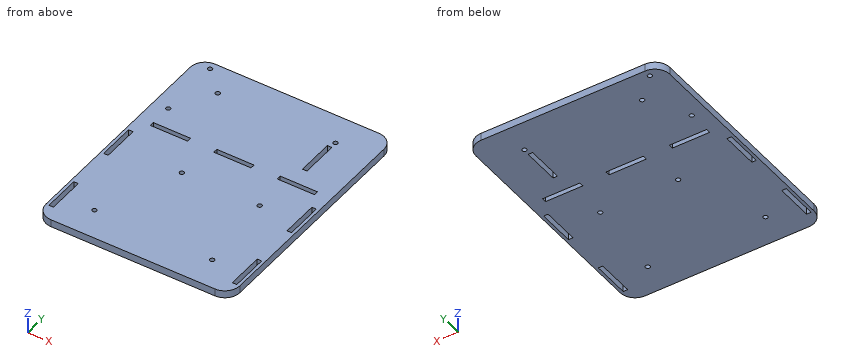
from build123d import *

# Parameters (mm, degrees)
RESSALTO_EXTRUS_O1_DEPTH = 5
ESBO_O2_R                = 1.5
CORTE_EXTRUS_O1_DEPTH    = 5
ESBO_O3_R                = 1.5
CORTE_EXTRUS_O2_DEPTH    = 6
ESBO_O6_W                = 3
ESBO_O6_H                = 25
ESBO_O6_W_2              = 25
ESBO_O6_H_2              = 3
CORTE_EXTRUS_O4_DEPTH    = 6
ESBO_O8_R                = 1.5
CORTE_EXTRUS_O6_DEPTH    = 10
ESBO_O9_W                = 3
ESBO_O9_H                = 25
CORTE_EXTRUS_O7_DEPTH    = 10


with BuildPart() as part:
    # Esboço1 → Ressalto-extrusão1 (new body)
    with BuildSketch(Plane.XY):
        with BuildLine():
            Line((-49.217119449, -36.393854661), (60.782880551, -36.393854661))
            ThreePointArc((60.782880551, -36.393854661), (67.853948363, -33.464922473), (70.782880551, -26.393854661))
            Line((70.782880551, -26.393854661), (70.782880551, 118.606145339))
            ThreePointArc((70.782880551, 118.606145339), (67.853948363, 125.67721315), (60.782880551, 128.606145339))
            Line((60.782880551, 128.606145339), (-49.217119449, 128.606145339))
            ThreePointArc((-49.217119449, 128.606145339), (-56.288187261, 125.67721315), (-59.217119449, 118.606145339))
            Line((-59.217119449, 118.606145339), (-59.217119449, -26.393854661))
            ThreePointArc((-59.217119449, -26.393854661), (-56.288187261, -33.464922473), (-49.217119449, -36.393854661))
        make_face()
    extrude(amount=RESSALTO_EXTRUS_O1_DEPTH)

    # Esboço2 → Corte-extrusão1 (cut)
    with BuildSketch(Plane(origin=(0, 0, 0), x_dir=(-1, 0, 0), z_dir=(0, 0, -1))):
        with Locations((33.717119449, -15.893854661)):
            Circle(ESBO_O2_R)
        with Locations((33.717119449, 108.106145339)):
            Circle(ESBO_O2_R)
        with Locations((-45.282880551, -15.893854661)):
            Circle(ESBO_O2_R)
        with Locations((-45.282880551, 108.106145339)):
            Circle(ESBO_O2_R)
    extrude(amount=-CORTE_EXTRUS_O1_DEPTH, mode=Mode.SUBTRACT)

    # Esboço3 → Corte-extrusão2 (cut, through all)
    with BuildSketch(Plane(origin=(0, 0, 0), x_dir=(-1, 0, 0), z_dir=(0, 0, -1))):
        with Locations((49.217119449, 123.606145339)):
            Circle(ESBO_O3_R)
        with Locations((49.217119449, 81.556145339)):
            Circle(ESBO_O3_R)
    extrude(amount=-CORTE_EXTRUS_O2_DEPTH, mode=Mode.SUBTRACT)

    # Esboço6 → Corte-extrusão4 (cut, through all)
    with BuildSketch(Plane(origin=(0, 0, 0), x_dir=(-1, 0, 0), z_dir=(0, 0, -1))):
        with Locations((-67.282880551, -13.893854661)):
            Rectangle(ESBO_O6_W, ESBO_O6_H)
        with Locations((-67.282880551, 41.106145339)):
            Rectangle(ESBO_O6_W, ESBO_O6_H)
        with Locations((-48.282880551, 65.106145339)):
            Rectangle(ESBO_O6_W_2, ESBO_O6_H_2)
        with Locations((36.717119449, 65.106145339)):
            Rectangle(ESBO_O6_W_2, ESBO_O6_H_2)
        with Locations((55.717119449, 41.106145339)):
            Rectangle(ESBO_O6_W, ESBO_O6_H)
        with Locations((55.717119449, -13.893854661)):
            Rectangle(ESBO_O6_W, ESBO_O6_H)
        with Locations((-5.782880551, 65.106145339)):
            Rectangle(ESBO_O6_W_2, ESBO_O6_H_2)
    extrude(amount=-CORTE_EXTRUS_O4_DEPTH, mode=Mode.SUBTRACT)

    # Esboço8 → Corte-extrusão6 (cut)
    with BuildSketch(Plane.XY.offset(5)):
        with Locations((-11.447119449, 38.606145339)):
            Circle(ESBO_O8_R)
        with Locations((40.782880551, 38.606145339)):
            Circle(ESBO_O8_R)
    extrude(amount=-CORTE_EXTRUS_O6_DEPTH, mode=Mode.SUBTRACT)

    # Esboço9 → Corte-extrusão7 (cut)
    with BuildSketch(Plane(origin=(0, 0, 0), x_dir=(-1, 0, 0), z_dir=(0, 0, -1))):
        with Locations((-44.282880551, 91.106145339)):
            Rectangle(ESBO_O9_W, ESBO_O9_H)
    extrude(amount=-CORTE_EXTRUS_O7_DEPTH, mode=Mode.SUBTRACT)


solid = part.part
Work out the finished part from the listing and answer in its coordinate system (mm). Round coordinates to 2 decimals unless told otherwise and drop trailing zeros. Write each loop counter-clockwise with the first axis right and the second up, starting at its lowest first coordinate (ties: lowest second). Pieces come first, ordered by that corner, then holes.
1) A cutting plane is placed at B-B (x = 0). Give the vertices of the cut face in (y, z), plus the area to 3 significant figures.
2) A cutting plane is placed at C-C (z = 2.85). Give the number of separate pieces and of enclosed holes in the cut face, plus the area to 3 significant figures.
3) Given pin 1 Ø0.9 at (x, z) = (68, 3.5) entering from +Y; pin 2 Ø2.5 at (x, z) = (67, 2.5) entering from -Y; pin 3 Ø2.5 at (x, z) = (66.5, 1.5) entering from -Y, each flat-ended and moving along its own axis, determine where each tip first touches the part or whether it passes through.
4) A cutting plane is placed at A-A (y = 48). Give the vertices of the cut face in (x, z), plus the area to 3 significant figures.
5) Straight lines are drawn through the part: line 1 (X direction, y = 51, z = 3.5); line 2 (Y direction, x = -11.5, z = 3.55); line 3 (X direction, y = 38.5, z = 3.45). For each, find the intervals that lie inside material, in ascending order.
Completed:
1. outline: (-36.39, 0) - (63.61, 0) - (63.61, 5) - (-36.39, 5) - close; (66.61, 0) - (128.61, 0) - (128.61, 5) - (66.61, 5) - close
1. area: 810 mm2
2. separate pieces: 1
2. enclosed holes: 16
2. area: 20,700 mm2
3. pin 1: stops at y = 125.97
3. pin 2: stops at y = -35.07
3. pin 3: stops at y = -35.34
4. outline: (-59.22, 0) - (-57.22, 0) - (-57.22, 5) - (-59.22, 5) - close; (-54.22, 0) - (65.78, 0) - (65.78, 5) - (-54.22, 5) - close; (68.78, 0) - (70.78, 0) - (70.78, 5) - (68.78, 5) - close
4. area: 620 mm2
5. line 1: x = -59.22 to -57.22, -54.22 to 65.78, 68.78 to 70.78
5. line 2: y = -36.39 to 37.11, 40.11 to 128.61
5. line 3: x = -59.22 to -57.22, -54.22 to -12.94, -9.95 to 39.29, 42.28 to 65.78, 68.78 to 70.78
